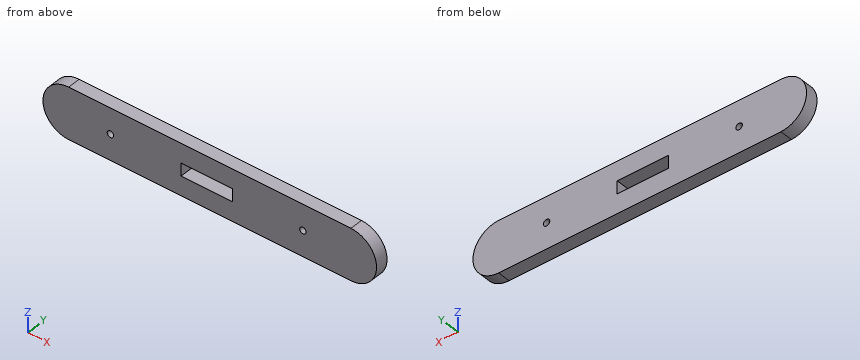
from build123d import *

# Parameters (mm, degrees)
SKETCH1_R           = 1.5875
SKETCH1_W           = 25.4
SKETCH1_H           = 6.35
BOSS_EXTRUDE1_DEPTH = 6.35


with BuildPart() as part:
    # Sketch1 → Boss-Extrude1 (new body)
    with BuildSketch(Plane(origin=(0, 0, 0), x_dir=(1, 0, 0), z_dir=(0, 1, 0))):
        with BuildLine():
            Line((72.335187692, -24.125963073), (-67.364812308, -24.125963073))
            ThreePointArc((-67.364812308, -24.125963073), (-80.064812308, -36.825963073), (-67.364812308, -49.525963073))
            Line((-67.364812308, -49.525963073), (72.335187692, -49.525963073))
            ThreePointArc((72.335187692, -49.525963073), (85.035187692, -36.825963073), (72.335187692, -24.125963073))
        make_face()
        with Locations(Location((-46.672412507, -36.825963073, 0), (0, 0, 270))):
            Circle(SKETCH1_R, mode=Mode.SUBTRACT)
        with Locations(Location((48.577587493, -36.825963073, 0), (0, 0, 270))):
            Circle(SKETCH1_R, mode=Mode.SUBTRACT)
        with Locations((0.952587493, -36.825963073)):
            Rectangle(SKETCH1_W, SKETCH1_H, mode=Mode.SUBTRACT)
    extrude(amount=BOSS_EXTRUDE1_DEPTH)


solid = part.part
The model under review builds one solid part; all positions refer to its coordinate system, in mm. Give positions to 0.01 mm unless a question says otherwise; leave off trailing zeros. Loops run counter-clockwise (first coordinate to the right, second up) from the corner with the lowest first, then second, coordinate; pieces in that order, holes last. Notation, with made-up numbers: (11, -34) -> (15, -34) arc R17 ccw to (15, -15) -> close; hole circle Ø7 at (73, 9). An arc over 180 degrees is marked (long way). Put each result on its own line as item: value. Start each with the question number.
1. We need section B-B on y = 4.75. State the section outline as (x, z) points (1 decimal).
2. Wall thickness on probe 1 along X at (y, z) = (5.5, 38.25); probe 2 along X at (y, z) = (1.25, 36); probe 3 along Z at (x, y) = (49.5, 1.75): over which ranges is each line inside the solid? List them lowest first.
3. Clearance check with a flat-ended pin moving along its axis: P1, Ø1, axis at y = 2, z = 41, coming from the -X side. State where the tip first meets the part, or that it passes through.
4. We need section A-A on x = -2. State the section outline as (y, z) points.
5. We need section D-D on z = 29.75. State the section outline as (x, y) points, then the cut area to 3 significant figures.
6. We need section C-C on z = 45.75. State the section outline as (x, y) points, then the cut area to 3 significant figures.
Determined:
1. outline: (-67.4, 24.1) -> (72.3, 24.1) arc R12.7 ccw to (72.3, 49.5) -> (-67.4, 49.5) arc R12.7 ccw to start; hole circle Ø3.2 at (-46.7, 36.8); hole (-11.7, 33.7) -> (13.7, 33.7) -> (13.7, 40) -> (-11.7, 40) -> close; hole circle Ø3.2 at (48.6, 36.8)
2. probe 1: -79.98 to -47.37, -45.97 to -11.75, 13.65 to 47.88, 49.28 to 84.96
2. probe 2: -80.04 to -48.03, -45.32 to -11.75, 13.65 to 47.22, 49.93 to 85.01
2. probe 3: 24.13 to 35.53, 38.12 to 49.53
3. P1: x = -79.52
4. outline: (0, 24.13) -> (6.35, 24.13) -> (6.35, 33.65) -> (0, 33.65) -> close; (0, 40) -> (6.35, 40) -> (6.35, 49.53) -> (0, 49.53) -> close
5. outline: (-77.91, 0) -> (82.88, 0) -> (82.88, 6.35) -> (-77.91, 6.35) -> close
5. area: 1,020 mm^2
6. outline: (-76.4, 0) -> (81.37, 0) -> (81.37, 6.35) -> (-76.4, 6.35) -> close
6. area: 1,000 mm^2
